from build123d import *

# Parameters (mm, degrees)
SKETCH1_R           = 9.8
SKETCH1_R_2         = 5
BOSS_EXTRUDE1_DEPTH = 10
SKETCH2_W           = 11.3
SKETCH2_H           = 11.3
CUT_EXTRUDE1_DEPTH  = 5
SKETCH3_W           = 11.313408722
SKETCH3_H           = 4.707055676
CUT_EXTRUDE2_DEPTH  = 3
SKETCH4_W           = 5.404805584
SKETCH4_H           = 18.076359344
SKETCH4_W_2         = 5.663408722
SKETCH4_H_2         = 17.947057775
CUT_EXTRUDE3_DEPTH  = 3
CHAMFER1_SIZE       = 3
SKETCH5_R           = 22.5
SKETCH5_R_2         = 9.8
BOSS_EXTRUDE2_DEPTH = 1
SKETCH6_R           = 11.25
SKETCH6_R_2         = 9.8
BOSS_EXTRUDE3_DEPTH = 5
SKETCH7_R           = 19.4
SKETCH7_R_2         = 18.75
BOSS_EXTRUDE4_DEPTH = 5
CHAMFER2_SIZE       = 0.25
SKETCH9_R           = 22.5
SKETCH9_R_2         = 9.8
BOSS_EXTRUDE5_DEPTH = 4
SKETCH10_W          = 11.313408722
SKETCH10_H          = 16.65
CUT_EXTRUDE5_DEPTH  = 3
CUT_EXTRUDE4_DEPTH  = 33.210246817
CIRPATTERN1_COUNT   = 6
SKETCH12_W          = 2.936696108
SKETCH12_H          = 13.215132487
SKETCH12_W_2        = 3.332020584
SKETCH12_H_2        = 13.328082337
BOSS_EXTRUDE6_DEPTH = 3
CHAMFER3_SIZE       = 1
CUT_EXTRUDE6_DEPTH  = 10
BOSS_EXTRUDE7_DEPTH = 2
BOSS_EXTRUDE8_DEPTH = 5
BOSS_EXTRUDE9_DEPTH = 5


with BuildPart() as part:
    # Sketch1 → Boss-Extrude1 (new body)
    with BuildSketch(Plane.XY):
        Circle(SKETCH1_R)
        Circle(SKETCH1_R_2, mode=Mode.SUBTRACT)
    extrude(amount=BOSS_EXTRUDE1_DEPTH)

    # Sketch2 → Cut-Extrude1 (cut)
    with BuildSketch(Plane.XY.offset(10)):
        Rectangle(SKETCH2_W, SKETCH2_H)
    extrude(amount=-CUT_EXTRUDE1_DEPTH, mode=Mode.SUBTRACT)

    # Sketch3 → Cut-Extrude2 (cut)
    with BuildSketch(Plane.XY.offset(10)):
        with Locations((0.006704361, 8.003527838)):
            Rectangle(SKETCH3_W, SKETCH3_H)
    extrude(amount=-CUT_EXTRUDE2_DEPTH, mode=Mode.SUBTRACT)

    # Sketch4 → Cut-Extrude3 (cut)
    with BuildSketch(Plane.XY.offset(10)):
        with Locations((-10.5897985, 0)):
            Rectangle(SKETCH4_W, SKETCH4_H)
        with Locations((10.615658814, 0.064650784)):
            Rectangle(SKETCH4_W_2, SKETCH4_H_2)
    extrude(amount=-CUT_EXTRUDE3_DEPTH, mode=Mode.SUBTRACT)

    # Chamfer1
    chamfer1_edges = [part.edges().sort_by_distance(p)[0] for p in [
        (-5, 0, 0),
    ]]
    chamfer(chamfer1_edges, length=CHAMFER1_SIZE)

    # Sketch5 → Boss-Extrude2 (add)
    with BuildSketch(Plane(origin=(0, 0, 5), x_dir=(-1, 0, 0), z_dir=(0, 0, -1))):
        Circle(SKETCH5_R)
        Circle(SKETCH5_R_2, mode=Mode.SUBTRACT)
    extrude(amount=-BOSS_EXTRUDE2_DEPTH)

    # Sketch6 → Boss-Extrude3 (add)
    with BuildSketch(Plane(origin=(0, 0, 5), x_dir=(-1, 0, 0), z_dir=(0, 0, -1))):
        with Locations(Location((0, 0, 0), (0, 0, 180))):
            Circle(SKETCH6_R)
        Circle(SKETCH6_R_2, mode=Mode.SUBTRACT)
    extrude(amount=BOSS_EXTRUDE3_DEPTH)

    # Sketch7 → Boss-Extrude4 (add)
    with BuildSketch(Plane(origin=(0, 0, 5), x_dir=(-1, 0, 0), z_dir=(0, 0, -1))):
        with Locations(Location((0, 0, 0), (0, 0, 180))):
            Circle(SKETCH7_R)
        with Locations(Location((0, 0, 0), (0, 0, 180))):
            Circle(SKETCH7_R_2, mode=Mode.SUBTRACT)
    extrude(amount=BOSS_EXTRUDE4_DEPTH)

    # Chamfer2
    chamfer2_edges = [part.edges().sort_by_distance(p)[0] for p in [
        (-19.4, 0, 0),
    ]]
    chamfer(chamfer2_edges, length=CHAMFER2_SIZE)

    # Sketch9 → Boss-Extrude5 (add)
    with BuildSketch(Plane.XY.offset(6)):
        with Locations(Location((0, 0, 0), (0, 0, 180))):
            Circle(SKETCH9_R)
        Circle(SKETCH9_R_2, mode=Mode.SUBTRACT)
    extrude(amount=BOSS_EXTRUDE5_DEPTH)

    # Sketch10 → Cut-Extrude5 (cut)
    with BuildSketch(Plane.XY.offset(10)):
        with Locations((0.006704361, 13.975)):
            Rectangle(SKETCH10_W, SKETCH10_H)
    extrude(amount=-CUT_EXTRUDE5_DEPTH, mode=Mode.SUBTRACT)

    # Sketch8 → Cut-Extrude4 (cut, through all)
    with BuildSketch(Plane(origin=(0, 0, 5), x_dir=(-1, 0, 0), z_dir=(0, 0, -1))):
        with BuildLine():
            Line((-7.732356662, 12.357593624), (1.172643737, 14.743669758))
            Line((1.172643737, 14.743669758), (0.137372224, 18.607374314))
            Line((0.137372224, 18.607374314), (-8.767628174, 16.22129818))
            ThreePointArc((-8.767628174, 16.22129818), (-10.181844696, 13.771810146), (-7.732356662, 12.357593624))
        make_face()
    cut_extrude4 = extrude(amount=-CUT_EXTRUDE4_DEPTH, mode=Mode.SUBTRACT)

    # CirPattern1: Cut-Extrude4 ×6 about axis
    cirpattern1_axis = Axis((0, 0, 0), (0, 0, 1))
    for i in range(1, CIRPATTERN1_COUNT):
        add(cut_extrude4.rotate(cirpattern1_axis, i * 360 / CIRPATTERN1_COUNT), mode=Mode.SUBTRACT)

    # Sketch12 → Boss-Extrude6 (add)
    with BuildSketch(Plane.XY.offset(7)):
        with Locations((-8.471238773, 0.2258997)):
            Rectangle(SKETCH12_W, SKETCH12_H)
        with Locations((8.555951161, 0.282374626)):
            Rectangle(SKETCH12_W_2, SKETCH12_H_2)
    extrude(amount=BOSS_EXTRUDE6_DEPTH)

    # Chamfer3
    chamfer3_edges = [part.edges().sort_by_distance(p)[0] for p in [
        (22.5, 0, 5),
    ]]
    chamfer(chamfer3_edges, length=CHAMFER3_SIZE)

    # Sketch13 → Cut-Extrude6 (cut)
    with BuildSketch(Plane.XY.offset(10)):
        Polygon((-16.183144966, 9.184719321), (-18.500019366, -1.9936e-05), (-14.638921299, 0.732314676), (-13.354714423, 6.356295613), align=None)
    extrude(amount=-CUT_EXTRUDE6_DEPTH, mode=Mode.SUBTRACT)

    # Sketch14 → Boss-Extrude7 (add)
    with BuildSketch(Plane.XY.offset(7)):
        Polygon((-0.137372224, 18.607374314), (5.663408722, 17.053067256), (5.663408722, 12.911963875), (-1.172643737, 14.743669758), align=None)
    extrude(amount=-BOSS_EXTRUDE7_DEPTH)

    # Sketch15 → Boss-Extrude8 (add)
    with BuildSketch(Plane.XY.offset(10)):
        with BuildLine():
            Line((8.767628174, 16.22129818), (5.663408722, 17.053067256))
            Line((5.663408722, 17.053067256), (5.663408722, 12.911963875))
            Line((5.663408722, 12.911963875), (7.732356662, 12.357593624))
            ThreePointArc((7.732356662, 12.357593624), (10.181844696, 13.771810146), (8.767628174, 16.22129818))
        make_face()
    extrude(amount=-BOSS_EXTRUDE8_DEPTH)

    # Sketch16 → Boss-Extrude9 (add)
    with BuildSketch(Plane.XY.offset(10)):
        with BuildLine():
            Line((-8.767628174, -16.22129818), (0.137372224, -18.607374314))
            Line((0.137372224, -18.607374314), (1.172643737, -14.743669758))
            Line((1.172643737, -14.743669758), (-7.732356662, -12.357593624))
            ThreePointArc((-7.732356662, -12.357593624), (-10.181844696, -13.771810146), (-8.767628174, -16.22129818))
        make_face()
    extrude(amount=-BOSS_EXTRUDE9_DEPTH)


solid = part.part
Part model, mm, in its own coordinate system. A direction names the side the tool comes from. Coordinates: 2 decimals unless noted, no trailing zeros. Write each question's results on one line, items separated by ' | '. Start each with the question number.
Q1. Which spindle directions (+Z, -Z, +X, -X, +Y, -Y) get a long thin tool onto all of the face, cutting with end or side? Do faces 5 (the flat face through (-12.97, 12.4, 7.46)), 6 (the flat face through (5.663, 14, 9)), 7 (the flat face through (5.65, 0, 8)), 8 (the flat face through (0, 22.3, 9)). Say none if no direction does.
Q2. Slice it at B-B on y = 0. Give the number of separate pieces and of enclosed holes in the cut face, and give its area (3 significant figures).
Q3. Drop flat-ended pins along their axis: pin 1 Ø4 at (y, z) = (11, 8.5) entering from -X; pin 2 Ø5.5 at (x, z) = (2, 6.5) entering from +Y; pin 3 Ø2.5 at (y, z) = (2, 8) entering from +X; pin 4 Ø6 at (x, y) = (0, 0) entering from -Z. Give the stop position or say it passes through.
Q4. Probe line 1 along Y through (x, z) = (0, 3.8); line 2 along Y through (x, z) = (15, 7.25); line 3 along X through (y, z) = (-5.5, 6.25). List the from-to ranges inside material, lowest first.
Q5. Two-plate mould, pull along Y, no slides. Class faces 1 (the flat face through (17.222, 5.032, 7.465)), 2 (the flat face through (0, -10, 10)), 3 (the cylindrical face through (-4.206, 18.939, 2.658)), 4 (the flat face through (9, -8, 5)): +Y half, -Y half, draft (parallel to the pull), parting line (faces both ways), or undercut.
Answer:
1) face 5: +Z, -Z | face 6: +Z, +Y | face 7: +Z | face 8: +Z, +X, -X
2) separate pieces: 4 | enclosed holes: 0 | area: 187 mm2
3) pin 1: stops at x = -20.62 | pin 2: stops at y = 22.5 | pin 3: stops at x = 22.49 | pin 4: passes through
4) line 1: y = -19.4 to -18.75, -11.25 to -5, 5 to 11.25, 18.75 to 19.4 | line 2: y = -16.77 to -10.37, -8 to -1.32, 9.14 to 16.77 | line 3: x = -21.82 to -17.1, -12.96 to -5.65, 5.65 to 21.82
5) face 1: undercut | face 2: draft | face 3: parting line | face 4: undercut
